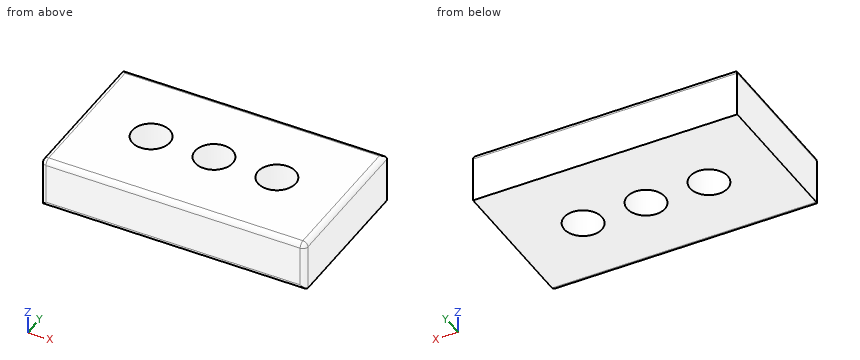
```python
from build123d import *

# Parameters (mm, degrees)
F0_W     = 266.7
F0_H     = 152.4
F0_R     = 19.05
F1_DEPTH = 50.8
F2_R     = 5.08


# Not quite as in the source:
# - a feature names something its author has since deleted; it is built from what else it names


with BuildPart() as f1:
    # F0 (on Top) → F1 (new body)
    with BuildSketch(Plane.XY):
        Rectangle(F0_W, F0_H)
        with Locations((-63.5, 0)):
            Circle(F0_R, mode=Mode.SUBTRACT)
        Circle(F0_R, mode=Mode.SUBTRACT)
        with Locations((63.5, 0)):
            Circle(F0_R, mode=Mode.SUBTRACT)
    extrude(amount=-F1_DEPTH)

    # F2
    f2_edges = [f1.edges().sort_by_distance(p)[0] for p in [
        (-133.35, 0, 0),
        (0, 76.2, 0),
        (133.35, 0, 0),
        (-133.35, -76.2, -25.4),
        (133.35, -76.2, -25.4),
        (0, -76.2, 0),
        (0, -76.2, -50.8),
    ]]
    fillet(f2_edges, radius=F2_R)


solid = f1.part
```
Could you check a few things on this model? Use its own coordinates, in mm. Round coordinates to 2 decimals unless told otherwise and drop trailing zeros. Loops run counter-clockwise (first coordinate to the right, second up) from the corner with the lowest first, then second, coordinate; pieces in that order, holes last.
Q1. I want a section at A-A (y = 0). Write out the boundary of the cut face in (x, z).
Q2. I want a section at B-B (x = 63.5). Write out the boundary of the cut face in (y, z), and give its area (3 significant figures).
Q3. I want a section at C-C (z = -39.5). Write out the boundary of the cut face in (x, y).
Q4. Please list where these lines run through material, in increasing order: L1, parallel to Y at x = 0, z = -27; L2, parallel to X at y = 4.5, z = -46.5; L3, parallel to Y at x = 30, z = -5.
Q5. I want a section at D-D (x = 15). Write out the boundary of the cut face in (y, z), and give its area (3 significant figures).
Q6. For P1, Ø23, axis at x = -63.5, y = 0, coming from the -Z side; P2, Ø5, axis at x = 9, y = 15, coming from the -Z side, each with a flat end and sliding along its axis, tell me the tip position at first contact or that it passes through.
Answer below:
1. outline: (-133.35, -50.8) - (-82.55, -50.8) - (-82.55, 0) - (-128.27, 0) arc R5.08 ccw to (-133.35, -5.08) - close; (-44.45, -50.8) - (-19.05, -50.8) - (-19.05, 0) - (-44.45, 0) - close; (19.05, -50.8) - (44.45, -50.8) - (44.45, 0) - (19.05, 0) - close; (82.55, -50.8) - (133.35, -50.8) - (133.35, -5.08) arc R5.08 ccw to (128.27, 0) - (82.55, 0) - close
2. outline: (-76.2, -45.72) arc R5.08 ccw to (-71.12, -50.8) - (-19.05, -50.8) - (-19.05, 0) - (-71.12, 0) arc R5.08 ccw to (-76.2, -5.08) - close; (19.05, -50.8) - (76.2, -50.8) - (76.2, -5.08) arc R5.08 ccw to (71.12, 0) - (19.05, 0) - close
2. area: 5,790 mm2
3. outline: (-133.35, -71.12) arc R5.08 ccw to (-128.27, -76.2) - (128.27, -76.2) arc R5.08 ccw to (133.35, -71.12) - (133.35, 76.2) - (-133.35, 76.2) - close; hole circle Ø38.1 at (-63.5, 0); hole circle Ø38.1 at (0, 0); hole circle Ø38.1 at (63.5, 0)
4. L1: y = -76.2 to -19.05, 19.05 to 76.2
4. L2: x = -133.35 to -82.01, -44.99 to -18.51, 18.51 to 44.99, 82.01 to 133.35
4. L3: y = -76.2 to 76.2
5. outline: (-76.2, -45.72) arc R5.08 ccw to (-71.12, -50.8) - (-11.74, -50.8) - (-11.74, 0) - (-71.12, 0) arc R5.08 ccw to (-76.2, -5.08) - close; (11.74, -50.8) - (76.2, -50.8) - (76.2, -5.08) arc R5.08 ccw to (71.12, 0) - (11.74, 0) - close
5. area: 6,530 mm2
6. P1: passes through
6. P2: stops at z = -50.8
